Read the model definition and answer for the solid it produces. Units are mm, in the model's axes. A direction names the side the tool comes from. Coordinates: 2 decimals unless noted, no trailing zeros. Order: outer loops, then holes, each group sorted by start corner. A loop starts at its lowest first (then second) coordinate and runs counter-clockwise, first axis right, second up. Notation, with made-up numbers: (87, 10.25) - (142, 10.25) arc R15 cw to (142, 19.25) - close; hole circle Ø6 at (-39, -5.75). An arc over 180 degrees is marked (long way). Write item = value, one per line.
from build123d import *

# Parameters (mm, degrees)
SKETCH1_R           = 7.5
BOSS_EXTRUDE1_DEPTH = 150
FILLET1_R           = 2
BOSS_EXTRUDE2_REACH = 129.5
SKETCH3_W           = 4.49
SKETCH3_H           = 6.99


with BuildPart() as part:
    # Sketch1 → Boss-Extrude1 (new body)
    with BuildSketch(Plane.XY):
        Circle(SKETCH1_R)
    extrude(amount=BOSS_EXTRUDE1_DEPTH)

    # Fillet1
    fillet1_edges = [part.edges().sort_by_distance(p)[0] for p in [
        (-7.5, 0, 0),
        (-7.5, 0, 150),
    ]]
    fillet(fillet1_edges, radius=FILLET1_R)

    # Sketch3 → Boss-Extrude2 (add, up to next)
    with BuildSketch(Plane(origin=(0, 120, 0), x_dir=(1, 0, 0), z_dir=(0, 1, 0)), mode=Mode.PRIVATE) as boss_extrude2_sk1:
        with Locations((0, -75)):
            Rectangle(SKETCH3_W, SKETCH3_H)
    boss_extrude2_tool1 = extrude(boss_extrude2_sk1.sketch, amount=-BOSS_EXTRUDE2_REACH, mode=Mode.PRIVATE) - part.part
    add(boss_extrude2_tool1.solids().sort_by_distance((0, 120, 75))[0])


solid = part.part
1) The part is cut by section A-A (x = 0). Determine the outline of the cut face in (y, z) (3 decimals).
Returned:
outline = (-7.5, 2) arc R2 ccw to (-5.5, 0) - (5.5, 0) arc R2 ccw to (7.5, 2) - (7.5, 71.505) - (120, 71.505) - (120, 78.495) - (7.5, 78.495) - (7.5, 148) arc R2 ccw to (5.5, 150) - (-5.5, 150) arc R2 ccw to (-7.5, 148) - close
2) Straight lines are drawn through the part: line 1 along Z through (x, y) = (-0.5, 49) (3 decimals); line 2 along Y through (x, z) = (0.5, 112.5); line 3 along Y through (x, z) = (-2.5, 72). For each, find the intervals that lie inside material, in ascending order. Write a range as from..to.
Returned:
line_1 = 71.505..78.495
line_2 = -7.48..7.48
line_3 = -7.07..7.07
3) The part is cut by section B-B (z = 42). Determine the outline of the cut face in (x, y).
Returned:
outline = circle Ø15 at (0, 0)
4) Flat-ended cylindrical pins translate along their axes: pin 1 Ø2 at (y, z) = (51, 73.5) entering from -X (3 decimals); pin 2 Ø4 at (x, z) = (-3, 94.5) entering from +Y; pin 3 Ø5 at (x, y) = (0, 106) entering from -Z (3 decimals). Find the tip coordinate at first contact, or state that the pin passes through.
Returned:
pin_1 = -2.245
pin_2 = 7.43
pin_3 = 71.505
5) The part is cut by section C-C (y = 108.5). Determine the outline of the cut face in (x, z) (3 decimals), and give its area (3 significant figures).
Returned:
outline = (-2.245, 71.505) - (2.245, 71.505) - (2.245, 78.495) - (-2.245, 78.495) - close
area = 31.4 mm^2
6) For faces 1 (the face through (0, 64, 78.495)), 2 (the face through (0, 64, 71.505)), 3 (the face through (2.245, 64, 75)), 4 (the face through (-2.245, 64, 75)), determine the directions among +Z, -Z, +X, -X, +Y, -Y from which every point of the face is accessible in a straight line to the end or side of a thin tool.
Returned:
face_1 = +Z, +X, -X, +Y
face_2 = -Z, +X, -X, +Y
face_3 = +Z, -Z, +X, +Y
face_4 = +Z, -Z, -X, +Y
